Geometry check sheet. Reference: the model listing, model coordinates, mm. A direction names the side the tool comes from. Give positions to 0.01 mm unless a question says otherwise; leave off trailing zeros. Loops run counter-clockwise (first coordinate to the right, second up) from the corner with the lowest first, then second, coordinate; pieces in that order, holes last. Notation, with made-up numbers: (83, 53.25) - (108, 53.25) arc R33 ccw to (108, 86.25) - close; hole circle Ø4 at (15.25, 42.25). An arc over 180 degrees is marked (long way). Use a Markdown table: item, result. Add a question column.
1. Cross-section at C-C on x = 33. Enter the section's corners in (y, z), and give its area (3 significant figures).
2. Material ranges on L1, parallel to Z at x = -42.5, y = -40.5; L2, parallel to Z at x = 39, y = -28; L3, parallel to X at y = -19, z = -8, recorded low to high.
3. Depth check by flat-ended pin: P1, Ø9.5, axis at x = -52.5, y = -44, coming from the +Z side; P2, Ø14, axis at x = 52.5, y = -45.5, coming from the -Z side; P3, Ø17, axis at x = 30, y = -56.5, coming from the -Z side. Enter the tip coordinate at first touch or a pass-through.
4. Set-up check for faces 1 (the flat face through (-50, -50, 0)), 2 (the flat face through (51, -50, -11.173)), 3 (the flat face through (30, -50, -2.939)): record each of +Z, -Z, +X, -X, +Y, -Y from which the full face is reachable in a straight line by a thin tool's end or side.
5. Cross-section at D-D on z = 8.5. Enter the section's corners in (x, y).
6. Draft check along X on faces 4 (the flat face through (-56.143, -50, -10)), 5 (the cylindrical face through (12.738, -50.089, -15.099)), 6 (the flat face through (0, 0, 0)), 7 (the flat face through (-32, -50, -3.187)). Enter one of: pulls with the +X half, pulls with the -X half, needs draft (parallel to the pull), parting line crosses it, or undercut.
7. Cross-section at B-B on z = -5. Enter the section's corners in (x, y), and give its area (3 significant figures).
8. Cross-section at A-A on y = -40. Enter the section's corners in (x, z).
from build123d import *

# Parameters (mm, degrees)
F1_DEPTH = 101.6


with BuildPart() as f1:
    # F0 (on Front) → F1 (new body)
    with BuildSketch(Plane.XZ):
        with BuildLine():
            ThreePointArc((0, -19.754416), (-12.792259, -15.053074), (-19.495674, -3.186789))
            Line((-19.495674, -3.186789), (-44.064047, -3.186789))
            Line((-44.064047, -3.186789), (-44.169664, 0))
            Line((-44.169664, 0), (-56.14337, 0))
            Line((-56.14337, 0), (-56.14337, -19.754416))
            Line((-56.14337, -19.754416), (0, -19.754416))
        make_face()
        with BuildLine():
            ThreePointArc((19.534622, -2.938621), (19.699391, -1.473415), (19.754416, 0))
            ThreePointArc((19.754416, 0), (13.968481, 13.968481), (0, 19.754416))
            ThreePointArc((0, 19.754416), (-15.053074, 12.792259), (-19.495674, -3.186789))
            ThreePointArc((-19.495674, -3.186789), (-12.792259, -15.053074), (0, -19.754416))
            ThreePointArc((0, -19.754416), (12.887711, -14.971434), (19.534622, -2.938621))
        make_face()
        with BuildLine():
            ThreePointArc((0, 19.754416), (13.968481, 13.968481), (19.754416, 0))
            ThreePointArc((19.754416, 0), (19.699391, -1.473415), (19.534622, -2.938621))
            Line((19.534622, -2.938621), (40.976677, -2.938621))
            Line((40.976677, -2.938621), (44.435747, -11.17319))
            Line((44.435747, -11.17319), (56.941614, -11.17319))
            Line((56.941614, -11.17319), (56.941614, 19.754416))
            Line((56.941614, 19.754416), (0, 19.754416))
        make_face()
    extrude(amount=F1_DEPTH)


solid = f1.part
Values found:
| question | item | result |
|---|---|---|
| 1 | outline | (-101.6, -2.94) - (0, -2.94) - (0, 19.75) - (-101.6, 19.75) - close |
| 1 | area | 2,310 mm2 |
| 2 | L1 | z = -19.75 to -3.19 |
| 2 | L2 | z = -2.94 to 19.75 |
| 2 | L3 | x = -56.14 to 18.06, 43.1 to 56.94 |
| 3 | P1 | stops at z = 0 |
| 3 | P2 | stops at z = -11.17 |
| 3 | P3 | stops at z = -2.94 |
| 4 | face 1 | +Z, -X, +Y, -Y |
| 4 | face 2 | -Z, +X, +Y, -Y |
| 4 | face 3 | -Z, +Y, -Y |
| 5 | outline | (-17.83, -101.6) - (56.94, -101.6) - (56.94, 0) - (-17.83, 0) - close |
| 6 | face 4 | pulls with the -X half |
| 6 | face 5 | undercut |
| 6 | face 6 | needs draft |
| 6 | face 7 | undercut |
| 7 | outline | (-56.14, -101.6) - (19.11, -101.6) - (19.11, 0) - (-56.14, 0) - close; (41.84, -101.6) - (56.94, -101.6) - (56.94, 0) - (41.84, 0) - close |
| 7 | area | 9,180 mm2 |
| 8 | outline | (-56.14, -19.75) - (0, -19.75) arc R19.75 ccw to (19.53, -2.94) - (40.98, -2.94) - (44.44, -11.17) - (56.94, -11.17) - (56.94, 19.75) - (0, 19.75) arc R19.75 ccw to (-19.5, -3.19) - (-44.06, -3.19) - (-44.17, 0) - (-56.14, 0) - close |
